Geometry check sheet. Reference: the model listing, model coordinates, mm. A direction names the side the tool comes from. Give positions to 0.01 mm unless a question says otherwise; leave off trailing zeros. Loops run counter-clockwise (first coordinate to the right, second up) from the corner with the lowest first, then second, coordinate; pieces in that order, holes last. Notation, with made-up numbers: (-9, 71.5) -> (48, 71.5) arc R27 cw to (48, 100.5) -> close; hole circle Ø2 at (22, -16.5). An arc over 180 degrees is marked (long way). Write item = value, one per line.
```python
from build123d import *

# Parameters (mm, degrees)
SKETCH_1_R               = 175
EXTRUDE_1_DEPTH          = 125
SHELL_3_T                = -5
SKETCH_2_W               = 5
SKETCH_2_H               = 105
CUT_REVOLVE_1_ANGLE      = 90
FILLET_1_R               = 10
FILLET_2_R               = 15
SKETCH_3_R               = 6.5
CUT_EXTRUDE_1_DEPTH      = 125
FILLET_3_R               = 10
FILLET_START             = 169
FILLET_4_DEPTH           = 7
SKETCH_5_R               = 4.5
CUT_EXTRUDE_2_DEPTH      = 125
PATTERN_CIRCULAR_1_COUNT = 3


with BuildPart() as part:
    # 草图1 → 凸台-拉伸1 (new body)
    with BuildSketch(Plane.XY):
        Circle(SKETCH_1_R)
    extrude(amount=EXTRUDE_1_DEPTH)

    # 抽壳3
    shell_3_openings = [part.faces().sort_by_distance(p)[0] for p in [
        (0, 0, 125),
    ]]
    offset(amount=SHELL_3_T, openings=shell_3_openings, kind=Kind.INTERSECTION)

    # 草图2 → 切除-旋转1 (revolve, cut)
    with BuildSketch(Plane(origin=(0, 0, 0), x_dir=(1, 0, 0), z_dir=(0, 1, 0))):
        with Locations((172.5, -72.5)):
            Rectangle(SKETCH_2_W, SKETCH_2_H)
    revolve(axis=Axis((0, 0, 0), (0, 0, 1)), revolution_arc=CUT_REVOLVE_1_ANGLE, mode=Mode.SUBTRACT)

    # 圆角1
    fillet_1_edges = [part.edges().sort_by_distance(p)[0] for p in [
        (-170, 0, 5),
    ]]
    fillet(fillet_1_edges, radius=FILLET_1_R)

    # 圆角2
    fillet_2_edges = [part.edges().sort_by_distance(p)[0] for p in [
        (-175, 0, 0),
    ]]
    fillet(fillet_2_edges, radius=FILLET_2_R)

    # 草图3 → 切除-拉伸1 (cut)
    with BuildSketch(Plane.XY.offset(5)):
        Circle(SKETCH_3_R)
    extrude(amount=-CUT_EXTRUDE_1_DEPTH, mode=Mode.SUBTRACT)

    # 圆角3
    fillet_3_edges = [part.edges().sort_by_distance(p)[0] for p in [
        (0, 172.5, 125),
    ]]
    fillet(fillet_3_edges, radius=FILLET_3_R)

    # 圆角4: read off the stored shape, not the designer's step
    # 圆角4 outline → 圆角4 (cut)
    with BuildSketch(Plane.YZ.offset(FILLET_START)):
        with BuildLine():
            ThreePointArc((-10, 125), (-2.928932188, 122.071067812), (0, 115))
            Line((0, 115), (0, 125))
            Line((0, 125), (-10, 125))
        make_face()
    extrude(amount=FILLET_4_DEPTH, mode=Mode.SUBTRACT)

    # 草图5 → 切除-拉伸2 (cut)
    with BuildSketch(Plane.XY.offset(5)):
        with Locations((-30.243552325, 17.616115995)):
            Circle(SKETCH_5_R)
    cut_extrude_2 = extrude(amount=-CUT_EXTRUDE_2_DEPTH, mode=Mode.SUBTRACT)

    # 阵列(圆周)1: 切除-拉伸2 ×3 about axis
    pattern_circular_1_axis = Axis((0, 0, 0), (0, 0, 1))
    for i in range(1, PATTERN_CIRCULAR_1_COUNT):
        add(cut_extrude_2.rotate(pattern_circular_1_axis, i * 360 / PATTERN_CIRCULAR_1_COUNT), mode=Mode.SUBTRACT)


solid = part.part
```
Item 1: Gauge pin test, flat ends, axial feed: pin 1 (4 mm diameter, centred on y = -18.5, z = 15.5, fed in from +X); pin 2 (5 mm diameter, centred on x = -129.5, z = 45.5, fed in from +Y); pin 3 (10 mm diameter, centred on y = -77.5, z = 38.5, fed in from +X). Record the tip position at first contact, or that the pin passes through.
Answer:
pin_1 = 174.22
pin_2 = 120.4
pin_3 = 159.28
Item 2: Draft check along Z on faces 4 (the flat face through (33, 2, 5)), 5 (the flat face through (33, 2, 0)), 6 (the cylindrical face through (34.67, 18.74, 2.54)). Enter one of: +Z half, -Z half, draft (parallel to the pull), parting line (faces both ways), or undercut.
Answer:
face_4 = +Z half
face_5 = -Z half
face_6 = draft
Item 3: Tool access check on faces 1 (the flat face through (120.32, 120.32, 20)), 2 (the cylindrical face through (1.942, -38.992, 2.535)), 3 (the cylindrical face through (-134.91, -103.44, 69.23)). Record the directions out of +Z, -Z, +X, -X, +Y, -Y that give a thin tool (end or side, any length) a straight path to the whole face; none if there is none.
Answer:
face_1 = +Z, +X, +Y
face_2 = +Z, -Z
face_3 = +Z
Item 4: Section check A-A, the plane z = 43. Record the cut outline in (x, y), plus the area to 3 significant figures.
Answer:
outline = (0, 170) -> (0, 175) arc R175 ccw (long way) to (175, 0) -> (170, 0) arc R170 cw (long way) to start
area = 4,060 mm^2
Item 5: Thickness scan on L1, parallel to X at y = -3.5, z = 27.5 (3 decimals); L2, parallel to X at y = -108, z = 9.5; L3, parallel to Y at x = -122, z = 88.5. Record the ranges inside material, lowest first. Write a range as [from, to].
Answer:
L1 = [-174.965, -169.964], [169.964, 174.965]
L2 = [-136.37, -129.14], [129.14, 136.37]
L3 = [-125.46, -118.39], [118.39, 125.46]
